```python
from build123d import *

# Parameters (mm, degrees)
SKETCH1_W               = 25.4
SKETCH1_H               = 50.8
SKETCH1_W_2             = 19.05
SKETCH1_H_2             = 44.45
BOSS_EXTRUDE1_DEPTH     = 215.9
CUT_EXTRUDE1_DEPTH      = 25.4
SKETCH3_R               = 2.5527
CUT_EXTRUDE2_DEPTH      = 25.4
CUT_EXTRUDE_THIN1_DEPTH = 26.4
SKETCH7_R               = 14.2875
CUT_EXTRUDE3_DEPTH      = 25.4


with BuildPart() as part:
    # Sketch1 → Boss-Extrude1 (new body)
    with BuildSketch(Plane.XY):
        with Locations((-12.7, 25.4)):
            Rectangle(SKETCH1_W, SKETCH1_H)
        with Locations((-12.7, 25.4)):
            Rectangle(SKETCH1_W_2, SKETCH1_H_2, mode=Mode.SUBTRACT)
    extrude(amount=BOSS_EXTRUDE1_DEPTH)

    # Sketch2 → Cut-Extrude1 (cut)
    with BuildSketch(Plane(origin=(0, 0, 0), x_dir=(0, 0, -1), z_dir=(1, 0, 0))):
        Polygon((0, 50.8), (-50.8, 0), (0, 0), align=None)
    extrude(amount=-CUT_EXTRUDE1_DEPTH, mode=Mode.SUBTRACT)

    # Sketch3 → Cut-Extrude2 (cut)
    with BuildSketch(Plane(origin=(0, 0, 0), x_dir=(0, 0, -1), z_dir=(1, 0, 0))):
        with Locations((-63.5, 38.1)):
            Circle(SKETCH3_R)
        with Locations((-63.5, 12.7)):
            Circle(SKETCH3_R)
        with Locations((-88.9, 25.4)):
            Circle(SKETCH3_R)
    extrude(amount=-CUT_EXTRUDE2_DEPTH, mode=Mode.SUBTRACT)

    # Sketch6 → Cut-Extrude-Thin1 (cut, through all)
    with BuildSketch(Plane(origin=(0, 0, 0), x_dir=(0, 0, -1), z_dir=(1, 0, 0))):
        with BuildLine():
            ThreePointArc((-190.5, 0), (-215.9, 25.4), (-190.5, 50.8))
            Line((-190.5, 50.8), (-190.5, 63.5))
            ThreePointArc((-190.5, 63.5), (-228.6, 25.4), (-190.5, -12.7))
            Line((-190.5, -12.7), (-190.5, 0))
        make_face()
    extrude(amount=-CUT_EXTRUDE_THIN1_DEPTH, mode=Mode.SUBTRACT)

    # Sketch7 → Cut-Extrude3 (cut)
    with BuildSketch(Plane(origin=(0, 0, 0), x_dir=(0, 0, -1), z_dir=(1, 0, 0))):
        with Locations((-190.5, 25.4)):
            Circle(SKETCH7_R)
    extrude(amount=-CUT_EXTRUDE3_DEPTH, mode=Mode.SUBTRACT)


solid = part.part
```
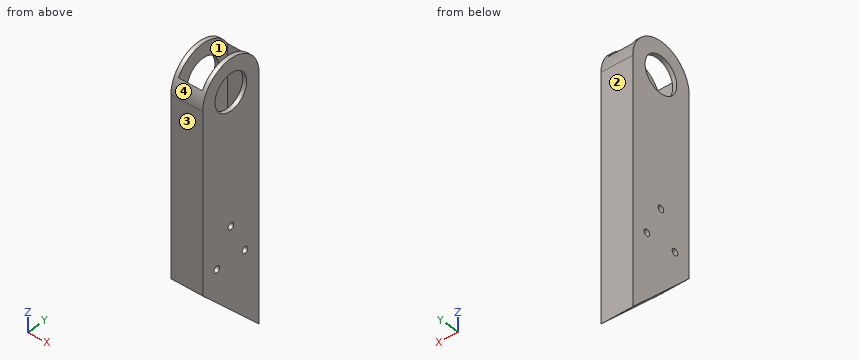
Read the model definition and answer for the solid it produces. Units are mm, in the model's axes. Face numbers are marked on the shaded views. Give positions to 0.01 mm unless a question says otherwise; leave off trailing zeros. Order: outer loops, then holes, each group sorted by start corner. A loop starts at its lowest first (then second) coordinate and runs counter-clockwise, first axis right, second up. Notation, with made-up numbers: (25, 51) -> (60, 51) arc R31 ccw to (60, 76) -> close; hole circle Ø1 at (76.5, 80). An arc over 180 degrees is marked (long way). One line per item, written item: value. Start each with the question number.
(1) The part is cut by section B-B (x = -5.75). Determine the outline of the cut face in (y, z) (3 decimals).
(2) The part is cut by section A-A (y = 25.4). Determine the outline of the cut face in (x, z) (1 decimal).
(3) The part is cut by section C-C (z = 88.9). Determine the outline of the cut face in (x, y) (3 decimals).
(4) Straight lines are drawn through the part: L1, parallel to X at y = 42.5, z = 34 (3 decimals); L2, parallel to Y at x = -6, z = 53 (3 decimals); L3, parallel to Y at x = -24.1, z = 88.9. For each, find the intervals that lie inside material, in ascending order.
(5) For a pull along Y with two mould halves and no side action, classify the marked faces 1, 2, 3 and 4 as released by +Y, released by -Y, zero draft, split by the parting line, or undercut.
(6) The part is cut by section D-D (z = 199.5). Determine the outline of the cut face in (x, y) (3 decimals).
(7) A flat-ended cylindrical pin translates along its axis: P1, Ø8, axis at y = 23.5, z = 78, coming from the +X side. Find the tip coordinate at first contact, or state that the pin passes through.
Taken from the geometry:
1. outline: (0, 50.8) -> (3.175, 47.625) -> (3.175, 202.797) arc R25.4 ccw to (0, 190.5) -> close; (47.625, 3.175) -> (50.8, 0) -> (50.8, 190.5) arc R25.4 ccw to (47.625, 202.797) -> close
2. outline: (-25.4, 25.4) -> (-22.2, 25.4) -> (-22.2, 86.3) -> (-25.4, 86.3) -> close; (-25.4, 91.5) -> (-22.2, 91.5) -> (-22.2, 176.2) -> (-25.4, 176.2) -> close; (-25.4, 204.8) -> (-22.2, 204.8) -> (-22.2, 215.9) -> (-25.4, 215.9) -> close; (-3.2, 25.4) -> (0, 25.4) -> (0, 86.3) -> (-3.2, 86.3) -> close; (-3.2, 91.5) -> (0, 91.5) -> (0, 176.2) -> (-3.2, 176.2) -> close; (-3.2, 204.8) -> (0, 204.8) -> (0, 215.9) -> (-3.2, 215.9) -> close
3. outline: (-25.4, 0) -> (0, 0) -> (0, 22.847) -> (-3.175, 22.847) -> (-3.175, 3.175) -> (-22.225, 3.175) -> (-22.225, 22.847) -> (-25.4, 22.847) -> close; (-25.4, 27.953) -> (-22.225, 27.953) -> (-22.225, 47.625) -> (-3.175, 47.625) -> (-3.175, 27.953) -> (0, 27.953) -> (0, 50.8) -> (-25.4, 50.8) -> close
4. L1: -25.4 to -22.225, -3.175 to 0
4. L2: 0 to 3.175, 47.625 to 50.8
4. L3: 0 to 22.85, 27.95 to 50.8
5. face 1: undercut
5. face 2: released by +Y
5. face 3: released by -Y
5. face 4: split by the parting line
6. outline: (-25.4, 1.648) -> (0, 1.648) -> (0, 14.303) -> (-3.175, 14.303) -> (-3.175, 3.175) -> (-22.225, 3.175) -> (-22.225, 14.303) -> (-25.4, 14.303) -> close; (-25.4, 36.497) -> (-22.225, 36.497) -> (-22.225, 47.625) -> (-3.175, 47.625) -> (-3.175, 36.497) -> (0, 36.497) -> (0, 49.152) -> (-25.4, 49.152) -> close
7. P1: x = 0
